```python
from build123d import *

# Parameters (mm, degrees)
SKETCH1_W           = 2.9
SKETCH1_H           = 4.25
SKETCH1_W_2         = 10
SKETCH1_H_2         = 3.2
BOSS_EXTRUDE1_DEPTH = 3.125
SKETCH3_W           = 71
SKETCH3_H           = 44.2
CUT_EXTRUDE1_DEPTH  = 3.125


with BuildPart() as part:
    # Sketch1 → Boss-Extrude1 (new body)
    with BuildSketch(Plane(origin=(0, 0, 0), x_dir=(1, 0, 0), z_dir=(0, 1, 0))):
        Polygon((-68.534526854, 15.117391304), (-52.534526854, 15.117391304), (-52.534526854, 25.117391304), (15.265473146, 25.117391304), (15.265473146, 15.117391304), (31.265473146, 15.117391304), (31.265473146, -36.882608696), (-68.534526854, -36.882608696), align=None)
        with Locations((-61.084526854, 2.367391304)):
            Rectangle(SKETCH1_W, SKETCH1_H, mode=Mode.SUBTRACT)
        with Locations((-61.084526854, -5.782608696)):
            Rectangle(SKETCH1_W, SKETCH1_H, mode=Mode.SUBTRACT)
        with Locations((-61.084526854, -13.932608696)):
            Rectangle(SKETCH1_W, SKETCH1_H, mode=Mode.SUBTRACT)
        with Locations((23.815473146, 2.367391304)):
            Rectangle(SKETCH1_W, SKETCH1_H, mode=Mode.SUBTRACT)
        with Locations((23.815473146, -5.782608696)):
            Rectangle(SKETCH1_W, SKETCH1_H, mode=Mode.SUBTRACT)
        with Locations((23.815473146, -13.932608696)):
            Rectangle(SKETCH1_W, SKETCH1_H, mode=Mode.SUBTRACT)
        with Locations((-36.834526854, 12.117391304)):
            Rectangle(SKETCH1_W_2, SKETCH1_H_2, mode=Mode.SUBTRACT)
        with Locations((-0.434526854, 12.117391304)):
            Rectangle(SKETCH1_W_2, SKETCH1_H_2, mode=Mode.SUBTRACT)
    extrude(amount=BOSS_EXTRUDE1_DEPTH)

    # Sketch3 → Cut-Extrude1 (cut)
    with BuildSketch(Plane(origin=(0, 3.125, 0), x_dir=(1, 0, 0), z_dir=(0, 1, 0))):
        with Locations((-18.634526854, -14.782608696)):
            Rectangle(SKETCH3_W, SKETCH3_H)
    extrude(amount=-CUT_EXTRUDE1_DEPTH, mode=Mode.SUBTRACT)


solid = part.part
```
CAD build for the part. Positions are in the model's coordinates, mm. A direction names the side the tool comes from. Round coordinates to 2 decimals unless told otherwise and drop trailing zeros. Order: outer loops, then holes, each group sorted by start corner. A loop starts at its lowest first (then second) coordinate and runs counter-clockwise, first axis right, second up.
Item 1: Saw through at C-C on z = 22.5. Write the cut outline in (x, y) (3 decimals), then the cut area to 3 significant figures.
Item 2: Saw through at D-D on y = 2.55. State how many separate pieces and enclosed holes the cut face has, then the cut area to 3 significant figures.
Item 3: Pin check, flat tip, straight feed: pin 1 (1.5 mm diameter, centred on x = -61.5, y = 1, fed in from -Z). Stop position of the tip, or through.
Item 4: Mould opens along X. For faces 4 (the face through (24, 2, 16.058)), 5 (the face through (24, 2, 36.883)), 6 (the face through (-68.535, 2, 11)), 7 (the face through (-59.635, 2, 6)) say: pulls with the +X half, pulls with the -X half, needs draft (parallel to the pull), parting line crosses it, or undercut.
Item 5: Probe line 1 along Z through (x, y) = (24, 1); line 2 along X through (y, z) = (2.95, -11); line 3 along X through (y, z) = (0.95, 12). List the from-to ranges inside material, lowest first.
Item 6: Saw through at A-A on z = 14. Write the cut outline in (x, y) (3 decimals), then the cut area to 3 significant figures.
Item 7: Tool access for faces 1 (the face through (16.865, 2, 15)), 2 (the face through (25.265, 2, 14)), 3 (the face through (15.265, 2, -20)): list every direction of +Z, -Z, +X, -X, +Y, -Y with a clear straight run to the whole face (end or side of a thin tool).
Item 8: Saw through at B-B on x = -37. Write the cut outline in (y, z) (3 decimals), then the cut area to 3 significant figures.
Reported:
1. outline: (-68.535, 0) - (-54.135, 0) - (-54.135, 3.125) - (-68.535, 3.125) - close; (16.865, 0) - (31.265, 0) - (31.265, 3.125) - (16.865, 3.125) - close
1. area: 90.0 mm2
2. separate pieces: 1
2. enclosed holes: 8
2. area: 2,590 mm2
3. pin 1: stops at z = -15.12
4. face 4: undercut
4. face 5: needs draft
4. face 6: pulls with the -X half
4. face 7: undercut
5. line 1: z = -15.12 to -4.49, -0.24 to 3.66, 7.91 to 11.81, 16.06 to 36.88
5. line 2: x = -68.53 to -41.83, -31.83 to -5.43, 4.57 to 31.27
5. line 3: x = -68.53 to -62.53, -59.63 to -54.13, 16.87 to 22.37, 25.27 to 31.27
6. outline: (-68.535, 0) - (-62.535, 0) - (-62.535, 3.125) - (-68.535, 3.125) - close; (-59.635, 0) - (-54.135, 0) - (-54.135, 3.125) - (-59.635, 3.125) - close; (16.865, 0) - (22.365, 0) - (22.365, 3.125) - (16.865, 3.125) - close; (25.265, 0) - (31.265, 0) - (31.265, 3.125) - (25.265, 3.125) - close
6. area: 71.9 mm2
7. face 1: +Z, +Y, -Y
7. face 2: +Y, -Y
7. face 3: -Z, +X, +Y, -Y
8. outline: (0, -25.117) - (3.125, -25.117) - (3.125, -13.717) - (0, -13.717) - close; (0, -10.517) - (3.125, -10.517) - (3.125, -7.317) - (0, -7.317) - close
8. area: 45.6 mm2
